Source: three-view drawing plus pictorial views. Frame: mm from the lowest corner of the part. A direction names the side the tool comes from. Give positions to 0.01 mm unless a question says otherwise; leave off trailing zeros. Order: outer loops, then holes, each group sorted by start corner. A loop starts at its lowest first (then second) coordinate and runs counter-clockwise, first axis right, second up. Notation, with made-up numbers: (89, 75.25) -> (144, 75.25) arc R24 ccw to (144, 88.25) -> close; hole circle Ø4 at (-30.5, 53.5). An arc over 180 degrees is marked (long way). Write item = value, one per line.
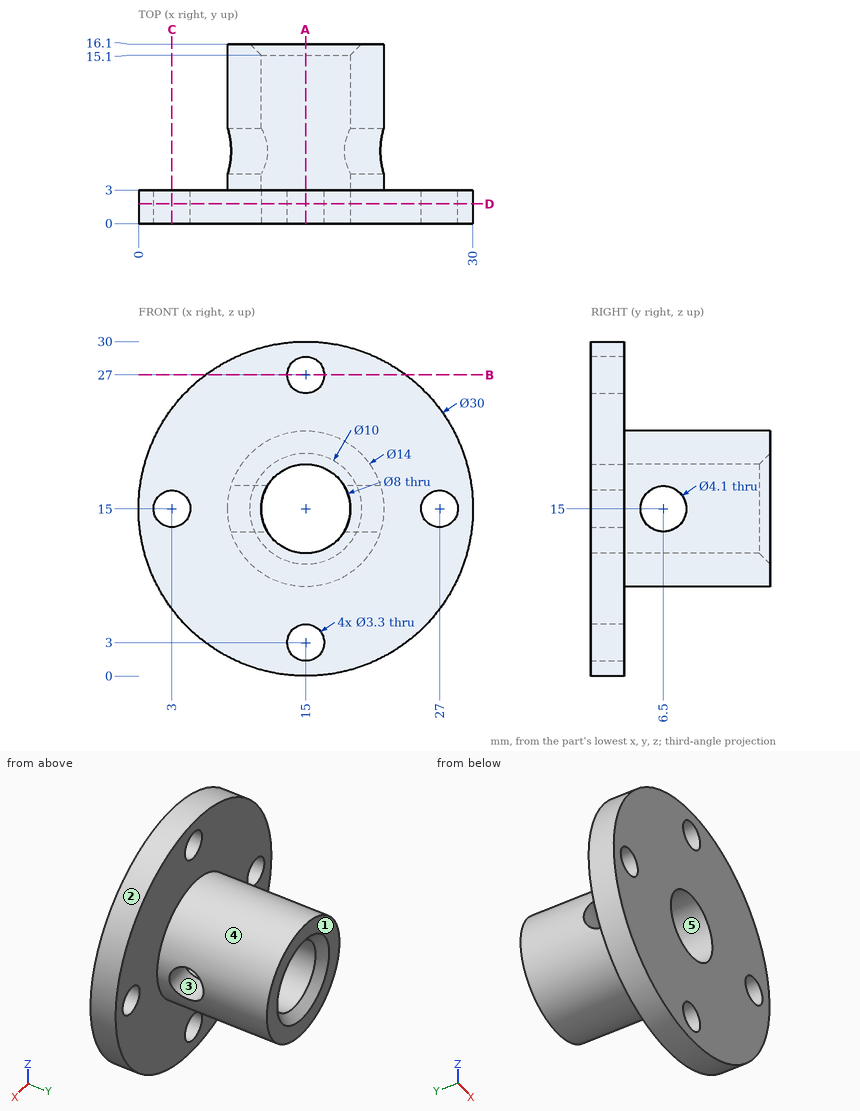
1) Section query B-B (z = 27). Output: boundary loops of the cut face in (x, y).
Check sheet entries:
outline = (6, 0) -> (13.35, 0) -> (13.35, 3) -> (6, 3) -> close; (16.65, 0) -> (24, 0) -> (24, 3) -> (16.65, 3) -> close
2) Section query C-C (x = 3). Output: boundary loops of the cut face in (y, z).
Check sheet entries:
outline = (0, 6) -> (3, 6) -> (3, 13.35) -> (0, 13.35) -> close; (0, 16.65) -> (3, 16.65) -> (3, 24) -> (0, 24) -> close
3) First-contact query: P1, Ø4.5, axis at x = 15, z = 3, coming from the +Y side; P2, Ø4, axis at y = 2.5, z = 22.5, coming from the -X side; P3, Ø4.5, axis at y = 6.5, z = 15, coming from the -X side; P4, Ø3, axis at x = 27, z = 15, coming from the -Y side. Flat tips, straight axial feed; report the tip coordinate or a pass-through.
Check sheet entries:
P1 = 3
P2 = 1.04
P3 = 8
P4 = through
4) Section query D-D (y = 1.75). Output: boundary loops of the cut face in (x, z), plus the area to 3 significant figures.
Check sheet entries:
outline = circle Ø30 at (15, 15); hole circle Ø3.3 at (3, 15); hole circle Ø8 at (15, 15); hole circle Ø3.3 at (15, 3); hole circle Ø3.3 at (15, 27); hole circle Ø3.3 at (27, 15)
area = 622 mm²
5) Mould query, pull axis Y, two halves, no side actions, for the marked faces 1, 2 and 3. Classes: +Y half, -Y half, draft (parallel to the pull), parting line (faces both ways), or undercut.
Check sheet entries:
face_1 = +Y half
face_2 = draft
face_3 = undercut
6) Section query A-A (x = 15). Output: boundary loops of the cut face in (y, z), plus the area to 3 significant figures.
Check sheet entries:
outline = (0, 0) -> (3, 0) -> (3, 1.35) -> (0, 1.35) -> close; (0, 4.65) -> (3, 4.65) -> (3, 8) -> (16.1, 8) -> (16.1, 10) -> (15.1, 11) -> (0, 11) -> close; (0, 19) -> (15.1, 19) -> (16.1, 20) -> (16.1, 22) -> (3, 22) -> (3, 25.35) -> (0, 25.35) -> close; (0, 28.65) -> (3, 28.65) -> (3, 30) -> (0, 30) -> close
area = 124 mm²
7) Line query: line 1 (X direction, y = 2.35, z = 15); line 2 (Z direction, x = 15, y = 7.25); line 3 (Y direction, x = 25.5, z = 20.5). Output: solid intervals per line, ascending. Write a range as from..to.
Check sheet entries:
line_1 = 0..1.35, 4.65..11, 19..25.35, 28.65..30
line_2 = 8..11, 19..22
line_3 = 0..3
8) Reachability of the marked faces 4 and 5 from +Z, -Z, +X, -X, +Y, -Y: full face, straight path, thin tool, end or side. Return the list, or none.
Check sheet entries:
face_4 = +Y
face_5 = +Y, -Y
